```python
from build123d import *

# Parameters (mm, degrees)
SKETCH_W        = 12.5
SKETCH_H        = 59
SKETCH_W_2      = 10
SKETCH_H_2      = 57
PAD_DEPTH       = 85
SKETCH001_W     = 12.5
SKETCH001_H     = 59
PAD001_DEPTH    = 2
POCKET_DEPTH    = 5
SKETCH003_W     = 20.915616
SKETCH003_H     = 3
POCKET001_DEPTH = 59.001


with BuildPart() as part:
    # Sketch → Pad (new body)
    with BuildSketch(Plane.XZ):
        with Locations((6.25, 29.5)):
            Rectangle(SKETCH_W, SKETCH_H)
        with Locations((6.5, 29.5)):
            Rectangle(SKETCH_W_2, SKETCH_H_2, mode=Mode.SUBTRACT)
    extrude(amount=PAD_DEPTH)

    # Sketch001 → Pad001 (new body)
    with BuildSketch(Plane.XZ.offset(85)):
        with Locations((6.25, 29.5)):
            Rectangle(SKETCH001_W, SKETCH001_H)
    extrude(amount=PAD001_DEPTH)

    # Sketch002 → Pocket (cut)
    with BuildSketch(Plane(origin=(0, 0, 0), x_dir=(0, 0, -1), z_dir=(-1, 0, 0))):
        with BuildLine():
            add(Edge.make_bspline(
                [(-29.5, -16), (-12.179492, -16), (-20.839746, 8), (-29.5, 32), (-38.160254, 8), (-46.820508, -16), (-29.5, -16)],
                knots=[0, 0, 0, 2.094395, 2.094395, 4.18879, 4.18879, 6.283185, 6.283185, 6.283185], degree=2, weights=[1, 0.5, 1, 0.5, 1, 0.5, 1]))
        make_face()
    extrude(amount=-POCKET_DEPTH, mode=Mode.SUBTRACT)

    # Sketch003 → Pocket001 (cut, through all)
    with BuildSketch(Plane(origin=(0, 0, 59), x_dir=(-1, 0, 0), z_dir=(0, 0, 1))):
        with Locations((-1.042192, 32.729344)):
            Rectangle(SKETCH003_W, SKETCH003_H)
    extrude(amount=-POCKET001_DEPTH, mode=Mode.SUBTRACT)


solid = part.part
```
Here's how the part is built. I have some questions about the finished solid (model axes, mm). A direction names the side the tool comes from. Coordinates: 2 decimals unless noted, no trailing zeros. Order: outer loops, then holes, each group sorted by start corner. A loop starts at its lowest first (then second) coordinate and runs counter-clockwise, first axis right, second up.
Item 1: I'm going to push flat-ended pins straight in: pin 1 Ø6 at (x, y) = (11, -60) entering from -Z; pin 2 Ø5 at (x, z) = (6.5, 43.5) entering from +Y. Where does each tip first touch, or does it pass through?
Response values:
pin 1: stops at z = 0
pin 2: stops at y = -85
Item 2: Which directions (+Z, -Z, +X, -X, +Y, -Y) give clear straight access to the entire face, cutting with the end or side of a thin tool? Please do faces 4 (the face through (6, -43, 0)), 5 (the face through (1, -34.229, 36)), 6 (the face through (6, -15, 58)).
Response values:
face 4: -Z, +X, -X, +Y, -Y
face 5: +Z, -Z, -X
face 6: +Y
Item 3: If we section it at B-B, the plane z = 50.5: List the corners of the cut face in (x, y) for me, then the cut area to 3 significant figures.
Response values:
outline: (0, -87) - (12.5, -87) - (12.5, 0) - (11.5, 0) - (11.5, -85) - (1.5, -85) - (1.5, -34.23) - (0, -34.23) - close; (0, -31.23) - (1.5, -31.23) - (1.5, 0) - (0, 0) - close
area: 233 mm2
Item 4: Thinking about a two-plate mould opening in Y: for faces 1 (the face through (1, -31.229, 36)), 2 (the face through (6, -87, 30)), 3 (the face through (6, -43, 59)), which applies, pulls with the +Y half, pulls with the -Y half, needs draft (parallel to the pull), parting line crosses it, or undercut?
Response values:
face 1: undercut
face 2: pulls with the -Y half
face 3: needs draft
Item 5: If we section it at C-C, the plane y = -74: List the corners of the cut face in (x, z) for me, then the cut area to 4 significant figures.
Response values:
outline: (0, 0) - (12.5, 0) - (12.5, 59) - (0, 59) - close; hole (1.5, 1) - (11.5, 1) - (11.5, 58) - (1.5, 58) - close
area: 167.5 mm2
Item 6: I need wall thicknesses on probe 1 along X at (y, z) = (-56.5, 5.5); probe 2 along Z at (x, y) = (3.5, -21); probe 3 along Y at (x, z) = (6, 41). Which ranges of each line are inside material? Lowest first, please.
Response values:
probe 1: x = 0 to 1.5, 11.5 to 12.5
probe 2: z = 0 to 1, 58 to 59
probe 3: y = -87 to -85
Item 7: If we section it at A-A, the plane x = 8.5: List the corners of the cut face in (y, z) for me, then the cut area to 3 significant figures.
Response values:
outline: (-87, 0) - (-34.23, 0) - (-34.23, 1) - (-85, 1) - (-85, 58) - (-34.23, 58) - (-34.23, 59) - (-87, 59) - close; (-31.23, 0) - (0, 0) - (0, 1) - (-31.23, 1) - close; (-31.23, 58) - (0, 58) - (0, 59) - (-31.23, 59) - close
area: 282 mm2
